Geometry check sheet. Reference: drawing and pictorial views, mm from the part's lowest x, y, z. Round coordinates to 2 decimals unless told otherwise and drop trailing zeros. Write each loop counter-clockwise with the first axis right and the second up, starting at its lowest first coordinate (ties: lowest second). Pieces come first, ordered by that corner, then holes. Notation, with made-up numbers: (-23.75, 76) -> (-1.75, 76) arc R37 ccw to (-1.75, 113) -> close; hole circle Ø8 at (-9, 28). An arc over 180 degrees is marked (long way). Write item = value, one per line.
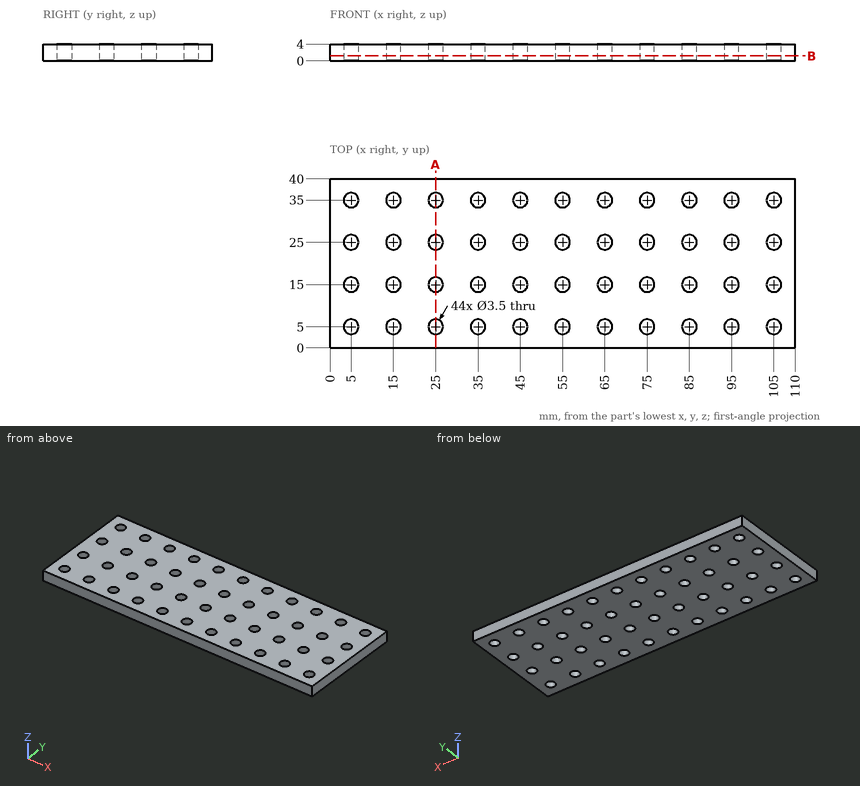
(1) Material ranges on L1, parallel to Y at x = 15, z = 1.6; L2, parallel to Y at x = 53.5, z = 2.55, recorded low to high. Write a range as [from, to].
Worked answers:
L1 = [0, 3.25], [6.75, 13.25], [16.75, 23.25], [26.75, 33.25], [36.75, 40]
L2 = [0, 4.1], [5.9, 14.1], [15.9, 24.1], [25.9, 34.1], [35.9, 40]
(2) Sectioned sample at B-B on z = 1.2. Count the separate pieces of the cut face and the enclosed holes in it, then the cut area to 3 significant figures.
Worked answers:
separate_pieces = 1
enclosed_holes = 44
area = 3,980 mm²
(3) Sectioned sample at A-A on x = 25. Enter the section's corners in (y, z), then the cut area to 3 significant figures.
Worked answers:
outline = (0, 0) -> (3.25, 0) -> (3.25, 4) -> (0, 4) -> close; (6.75, 0) -> (13.25, 0) -> (13.25, 4) -> (6.75, 4) -> close; (16.75, 0) -> (23.25, 0) -> (23.25, 4) -> (16.75, 4) -> close; (26.75, 0) -> (33.25, 0) -> (33.25, 4) -> (26.75, 4) -> close; (36.75, 0) -> (40, 0) -> (40, 4) -> (36.75, 4) -> close
area = 104 mm²
